Design review of the part built by this model. Coordinates are the model's own, in mm. Coordinates: 2 decimals unless noted, no trailing zeros. Write each loop counter-clockwise with the first axis right and the second up, starting at its lowest first coordinate (ties: lowest second). Pieces come first, ordered by that corner, then holes. Notation, with made-up numbers: (-23, 4.5) -> (3, 4.5) arc R11 cw to (3, 18.5) -> close; hole circle Ø1 at (43, -8.75). An arc over 180 degrees is marked (long way). Return JSON: item names as keys, results as strings. Group by question number.
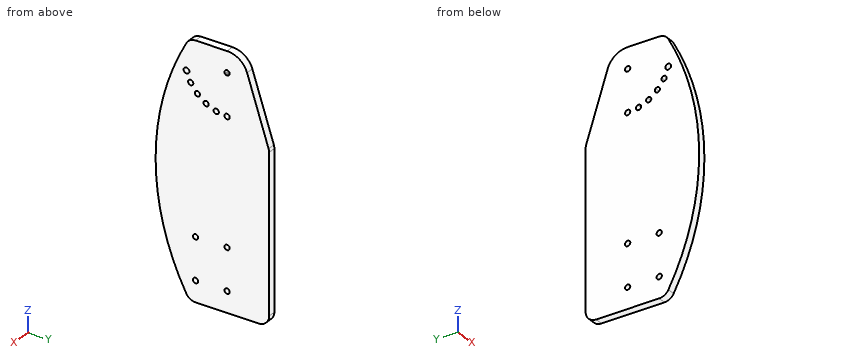
from build123d import *

# Parameters (mm, degrees)
F0_R     = 6.35
F0_R_2   = 7.002019
F1_DEPTH = 19.05
F3_DEPTH = 19.051


with BuildPart() as f1:
    # F0 (on Right) → F1 (new body)
    with BuildSketch(Plane.YZ):
        with BuildLine():
            ThreePointArc((-19.946015, 155.861936), (-21.258221, 159.727571), (-24.652514, 161.995565))
            ThreePointArc((-24.652514, 161.995565), (-31.333809, 151.996301), (-19.946015, 155.861936))
        make_face()
        with BuildLine():
            ThreePointArc((-44.45, 166.011819), (-45.300739, 169.186819), (-47.625, 171.51108))
            ThreePointArc((-47.625, 171.51108), (-56.299261, 162.836819), (-44.45, 166.011819))
        make_face()
        with BuildLine():
            ThreePointArc((-65.492049, 182.157951), (-65.975414, 184.587991), (-67.351921, 186.648079))
            ThreePointArc((-67.351921, 186.648079), (-77.708684, 179.727911), (-65.492049, 182.157951))
        make_face()
        with BuildLine():
            ThreePointArc((-81.638181, 203.2), (-81.854552, 204.843501), (-82.48892, 206.375))
            ThreePointArc((-82.48892, 206.375), (-94.12181, 201.556499), (-81.638181, 203.2))
        make_face()
        with BuildLine():
            Line((-76.2, -304.8), (76.2, -304.8))
            ThreePointArc((76.2, -304.8), (94.160512, -297.360512), (101.6, -279.4))
            Line((101.6, -279.4), (101.6, 304.8))
            Line((101.6, 304.8), (-76.2, 304.8))
            ThreePointArc((-76.2, 304.8), (-89.17315, 301.237065), (-98.506733, 291.547826))
            ThreePointArc((-98.506733, 291.547826), (-172.745149, 0), (-98.506733, -291.547826))
            ThreePointArc((-98.506733, -291.547826), (-89.17315, -301.237065), (-76.2, -304.8))
        make_face()
        with Locations((-76.2, -254)):
            Circle(F0_R, mode=Mode.SUBTRACT)
        with Locations((-76.2, -152.4)):
            Circle(F0_R, mode=Mode.SUBTRACT)
        with Locations((0, -254)):
            Circle(F0_R, mode=Mode.SUBTRACT)
        with Locations((0, -152.4)):
            Circle(F0_R, mode=Mode.SUBTRACT)
        with BuildLine():
            ThreePointArc((-65.492049, 182.157951), (-77.708684, 179.727911), (-67.351921, 186.648079))
            ThreePointArc((-67.351921, 186.648079), (-65.975414, 184.587991), (-65.492049, 182.157951))
        make_face(mode=Mode.SUBTRACT)
        with BuildLine():
            ThreePointArc((-81.638181, 203.2), (-94.12181, 201.556499), (-82.48892, 206.375))
            ThreePointArc((-82.48892, 206.375), (-81.854552, 204.843501), (-81.638181, 203.2))
        make_face(mode=Mode.SUBTRACT)
        with Locations((-98.138064, 227.703985)):
            Circle(F0_R_2, mode=Mode.SUBTRACT)
        with BuildLine():
            ThreePointArc((-44.45, 166.011819), (-56.299261, 162.836819), (-47.625, 171.51108))
            ThreePointArc((-47.625, 171.51108), (-45.300739, 169.186819), (-44.45, 166.011819))
        make_face(mode=Mode.SUBTRACT)
        with Locations((0, 152.4)):
            Circle(F0_R, mode=Mode.SUBTRACT)
        with BuildLine():
            ThreePointArc((-19.946015, 155.861936), (-31.333809, 151.996301), (-24.652514, 161.995565))
            ThreePointArc((-24.652514, 161.995565), (-21.258221, 159.727571), (-19.946015, 155.861936))
        make_face(mode=Mode.SUBTRACT)
        with BuildLine():
            ThreePointArc((-5.499261, 250.825), (-1.643501, 260.133629), (6.35, 254))
            ThreePointArc((6.35, 254), (3.865635, 248.962206), (-1.643501, 247.866371))
            ThreePointArc((-1.643501, 247.866371), (-2.43004, 248.133365), (-3.175, 248.500739))
            ThreePointArc((-3.175, 248.500739), (-3.865635, 248.962206), (-4.490128, 249.509872))
            ThreePointArc((-4.490128, 249.509872), (-5.037794, 250.134365), (-5.499261, 250.825))
        make_face(mode=Mode.SUBTRACT)
    extrude(amount=F1_DEPTH)

    # F2 (on face) → F3 (cut, through all)
    with BuildSketch(Plane(origin=(0, 0, 0), x_dir=(0, -1, 0), z_dir=(-1, 0, 0))):
        with BuildLine():
            ThreePointArc((-48.315877, 269.691272), (-29.862379, 295.095965), (0, 304.8))
            Line((0, 304.8), (-101.6, 304.8))
            Line((-101.6, 304.8), (-101.6, 101.6))
            ThreePointArc((-101.6, 101.6), (-101.287563, 105.571672), (-100.357939, 109.445636))
            Line((-100.357939, 109.445636), (-48.315877, 269.691272))
        make_face()
    extrude(amount=-F3_DEPTH, mode=Mode.SUBTRACT)


solid = f1.part
Q1. We need section C-C on z = 118.5. Write out the cut boundary in (x, y), plus the area to 3 significant figures.
Q2. Wall thickness on L1, parallel to Z at x = 7.75, y = 0; L2, parallel to Z at x = 8, y = -50.8; L3, parallel to Z at x = 13.75, y = -76.2: over which ranges is each line inside the solid? List them lowest first.
Q3. We need section A-A on x = 10. State how many separate pieces and enclosed holes the cut face has, plus the area to 3 significant figures.
Q4. For P1, Ø16.5, axis at y = 0, z = -254, coming from the -X side; P2, Ø1.5, axis at x = 16.5, z = -39, coming from the -Y side, all flat-tipped, find the tip position at first contact; note any pin that passes through.
Q5. We need section D-D on z = -225. Write out the cut boundary in (x, y), plus the area to 3 significant figures.
Q6. We need section B-B on z = -152.4. Write out the cut boundary in (x, y), plus the area to 3 significant figures.
Findings below:
{
 "1": {"outline": "(0, -161.12) -> (19.05, -161.12) -> (19.05, 97.42) -> (0, 97.42) -> close", "area": "4,930 mm^2"},
 "2": {"L1": "z = -304.8 to -260.35, -247.65 to -158.75, -146.05 to 146.05, 158.75 to 247.65, 260.35 to 304.8", "L2": "z = -304.8 to 159.66, 172.36 to 304.8", "L3": "z = -304.8 to -260.35, -247.65 to -158.75, -146.05 to 177.54, 186.78 to 304.8"},
 "3": {"separate pieces": "1", "enclosed holes": "11", "area": "143,000 mm^2"},
 "4": {"P1": "stops at x = 0", "P2": "stops at y = -171.54"},
 "5": {"outline": "(0, -129.7) -> (19.05, -129.7) -> (19.05, 101.6) -> (0, 101.6) -> close", "area": "4,410 mm^2"},
 "6": {"outline": "(0, -153.39) -> (19.05, -153.39) -> (19.05, -82.55) -> (0, -82.55) -> close; (0, -69.85) -> (19.05, -69.85) -> (19.05, -6.35) -> (0, -6.35) -> close; (0, 6.35) -> (19.05, 6.35) -> (19.05, 101.6) -> (0, 101.6) -> close", "area": "4,370 mm^2"}
}
